Design review of the part shown in the three views and the two pictorial views. Dimensions are in mm from the part's minimum x, y and z. A direction names the side the tool comes from. Give positions to 0.01 mm unless a question says otherwise; leave off trailing zeros. Order: outer loops, then holes, each group sorted by start corner. A loop starts at its lowest first (then second) coordinate and runs counter-clockwise, first axis right, second up. Notation, with made-up numbers: (79, -20) -> (101, -20) arc R13 ccw to (101, -16) -> close; hole circle Ø4 at (-18, -18.5). An arc over 180 degrees is marked (long way). Answer in a Markdown table with one row per item. Add a question column.
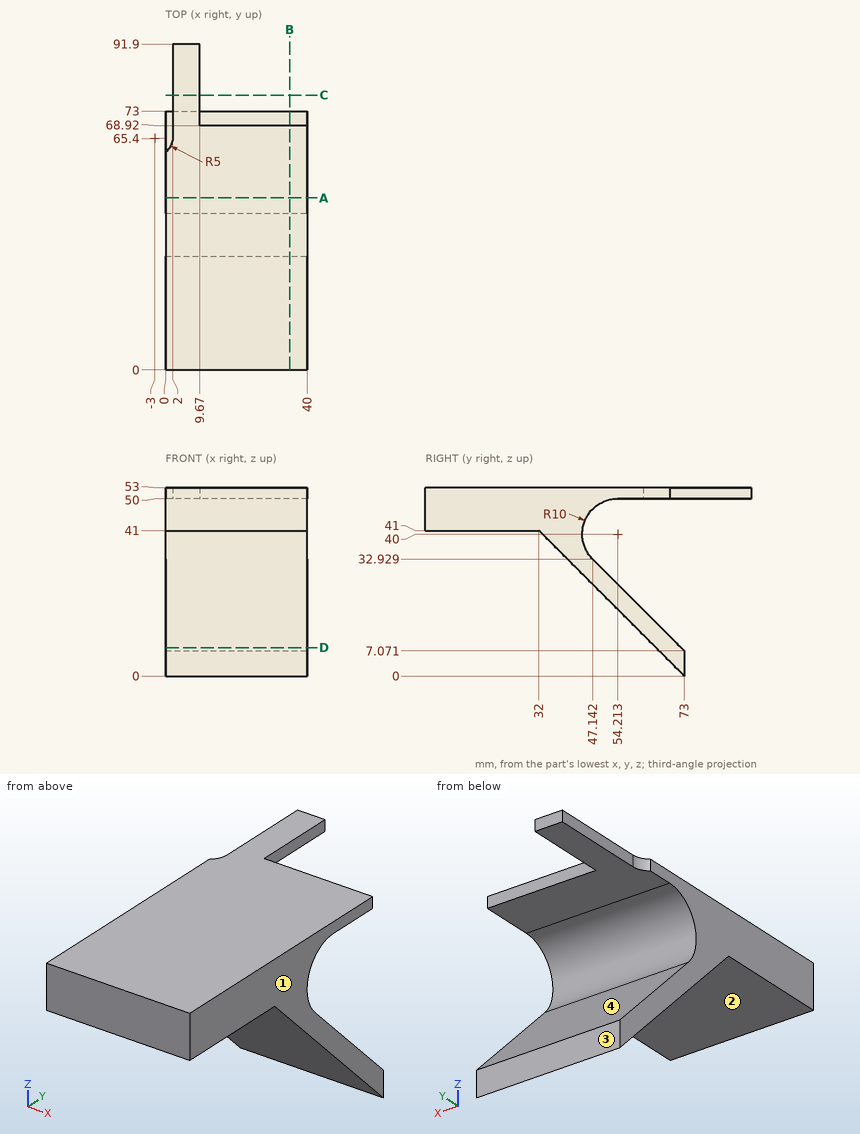
1) Add section B-B, the plane x = 35. Write out the cut boundary in (y, z).
2) For L1, parallel to Z at x = 34.5, y = 25.5; L2, parallel to Z at x = 17, y = 60; L3, parallel to Z at x = 13, y = 58.5, list the stretches that pass through material, from the lowest coordinate up.
3) Machinability: for the marked faces 1, 2, 3 and 4, which of the approach directions +Z, -Z, +X, -X, +Y, -Y give a long, thin tool a straight path to every point of the face, cutting with its end or side? Answer none if there is none.
4) Clearance check with flat-ended pins moving along their axes: P1, Ø1.5, axis at x = 28.5, z = 51.5, coming from the +Y side; P2, Ø1.5, axis at y = 80.5, z = 51, coming from the -X side; P3, Ø4, axis at y = 14, z = 37.5, coming from the +X side; P4, Ø2.5, axis at y = 78.5, z = 52, coming from the +X side. State where each tip first meets the part, or that it passes through.
5) Add section D-D, the plane z = 8. Write out the cut boundary in (x, y).
6) Add section A-A, the plane y = 48.5. Write out the cut boundary in (x, z).
7) Add section C-C, the plane y = 77.5. Write out the cut boundary in (x, z), and give its area (3 significant figures).
Verdict:
| question | item | result |
|---|---|---|
| 1 | outline | (0, 41) -> (32, 41) -> (73, 0) -> (73, 7.07) -> (47.14, 32.93) arc R10 cw to (54.21, 50) -> (68.92, 50) -> (68.92, 53) -> (0, 53) -> close |
| 2 | L1 | z = 41 to 53 |
| 2 | L2 | z = 13 to 20.07, 50 to 53 |
| 2 | L3 | z = 14.5 to 21.57, 50 to 53 |
| 3 | face 1 | +Z, -Z, +X, +Y, -Y |
| 3 | face 2 | -Z, +X, -X, -Y |
| 3 | face 3 | -Z, +X, -X, +Y |
| 3 | face 4 | +X, -X, +Y |
| 4 | P1 | stops at y = 68.92 |
| 4 | P2 | stops at x = 2 |
| 4 | P3 | passes through |
| 4 | P4 | stops at x = 9.67 |
| 5 | outline | (0, 65) -> (40, 65) -> (40, 72.07) -> (0, 72.07) -> close |
| 6 | outline | (0, 24.5) -> (40, 24.5) -> (40, 31.57) -> (0, 31.57) -> close; (0, 48.21) -> (40, 48.21) -> (40, 53) -> (0, 53) -> close |
| 7 | outline | (2, 50) -> (9.67, 50) -> (9.67, 53) -> (2, 53) -> close |
| 7 | area | 23.0 mm2 |
